```python
from build123d import *

# Parameters (mm, degrees)
SKETCH1_R           = 22.6
SKETCH1_R_2         = 6
BOSS_EXTRUDE1_DEPTH = 6
CUT_EXTRUDE1_DEPTH  = 6
CIRPATTERN1_COUNT   = 15


with BuildPart() as part:
    # Sketch1 → Boss-Extrude1 (new body)
    with BuildSketch(Plane(origin=(0, 0, 0), x_dir=(0, 0, -1), z_dir=(1, 0, 0))):
        Circle(SKETCH1_R)
        Circle(SKETCH1_R_2, mode=Mode.SUBTRACT)
    extrude(amount=BOSS_EXTRUDE1_DEPTH)

    # Sketch2 → Cut-Extrude1 (cut)
    with BuildSketch(Plane(origin=(6, 0, 0), x_dir=(0, 0, -1), z_dir=(1, 0, 0))):
        with BuildLine():
            Line((-3.5, 22.327337504), (-1.808436926, 18.745859565))
            ThreePointArc((-1.808436926, 18.745859565), (0, 17.6), (1.808436926, 18.745859565))
            Line((1.808436926, 18.745859565), (3.5, 22.327337504))
            Line((3.5, 22.327337504), (0, 25.827337504))
            Line((0, 25.827337504), (-3.5, 22.327337504))
        make_face()
    cut_extrude1 = extrude(amount=-CUT_EXTRUDE1_DEPTH, mode=Mode.SUBTRACT)

    # CirPattern1: Cut-Extrude1 ×15 about axis
    cirpattern1_axis = Axis((0, 0, 0), (1, 0, 0))
    for i in range(1, CIRPATTERN1_COUNT):
        add(cut_extrude1.rotate(cirpattern1_axis, i * 360 / CIRPATTERN1_COUNT), mode=Mode.SUBTRACT)


solid = part.part
```
Verification items for the finished model (mm, model axes). A direction names the side the tool comes from. Coordinates: 2 decimals unless noted, no trailing zeros. Write each loop counter-clockwise with the first axis right and the second up, starting at its lowest first coordinate (ties: lowest second). Pieces come first, ordered by that corner, then holes. Notation, with made-up numbers: M -40,-28.75 L -9,-28.75 A17 cw -9,-13.75 Z; hole C -3,-40 d11. An arc over 180 degrees is marked long. One line per item, written item: value.
Item 1: Section check C-C, the plane z = 7.5. Record the boundary of the cut face in (x, y), plus the area to 3 significant figures.
Check sheet entries:
outline: M 0,-20.37 L 6,-20.37 L 6,15.96 L 0,15.96 Z
area: 218 mm^2
Item 2: Access from +Z, -Z, +X, -X, +Y, -Y to the whole of each face (thin tool, end or side, straight path). Record for faces 5 (the flat face through (3.04, 8.89, -18.73)), 6 (the flat face through (3.04, 20.51, -2.64)), 7 (the flat face through (3.04, -15.04, 14.19)), 8 (the flat face through (3.042, -12.59, 16.474)).
Check sheet entries:
face 5: -Z, +X, -X
face 6: +X, -X, +Y
face 7: +X, -X, -Y
face 8: +Z, +X, -X
Item 3: Section check A-A, the plane z = 0. Record the boundary of the cut face in (x, y), plus the area to 3 significant figures.
Check sheet entries:
outline: M 0,-22.6 L 6,-22.6 L 6,-6 L 0,-6 Z; M 0,6 L 6,6 L 6,17.6 L 0,17.6 Z
area: 169 mm^2
Item 4: Section check B-B, the plane y = 2.5. Record the boundary of the cut face in (x, z), plus the area to 3 significant figures.
Check sheet entries:
outline: M 0,-22.46 L 6,-22.46 L 6,-5.45 L 0,-5.45 Z; M 0,5.45 L 6,5.45 L 6,22.46 L 0,22.46 Z
area: 204 mm^2
Item 5: Gauge pin test, flat ends, axial feed: pin 1 Ø2 at (x, z) = (4.5, -5) entering from -Y; pin 2 Ø1.5 at (x, y) = (3.5, 12.5) entering from -Z; pin 3 Ø2 at (x, z) = (3.5, -15.5) entering from +Y. Record the tip position at first contact, or that the pin passes through.
Check sheet entries:
pin 1: stops at y = -18.4
pin 2: stops at z = -19.31
pin 3: stops at y = 11.61
Item 6: Mould release check, pull along Z, two halves, no side actions. Record for faces 1 (the cylindrical face through (3.04, 16.09, -7.13)), 2 (the cylindrical face through (3, -22.6, 0)), 3 (the cylindrical face through (2.96, 22.11, 4.68)), 4 (the cylindrical face through (2.96, -7, -21.49)): pulls with the +Z half, pulls with the -Z half, needs draft (parallel to the pull), parting line crosses it, or undercut.
Check sheet entries:
face 1: undercut
face 2: parting line crosses it
face 3: pulls with the +Z half
face 4: pulls with the -Z half
Item 7: Scan lines: line 1 along Y through (x, z) = (5.15, -18.5); line 2 along Z through (x, y) = (3.9, 16.5); line 3 along Y through (x, z) = (1.1, -16). Record each from-to range of solid material in increasing order.
Check sheet entries:
line 1: y = -7.92 to -3.79, -0.31 to 4.06, 8.67 to 12.21
line 2: z = -13.81 to -9.4, -6.55 to 6.55, 9.4 to 13.81
line 3: y = -15.96 to -11.91, -8.05 to 11.46
